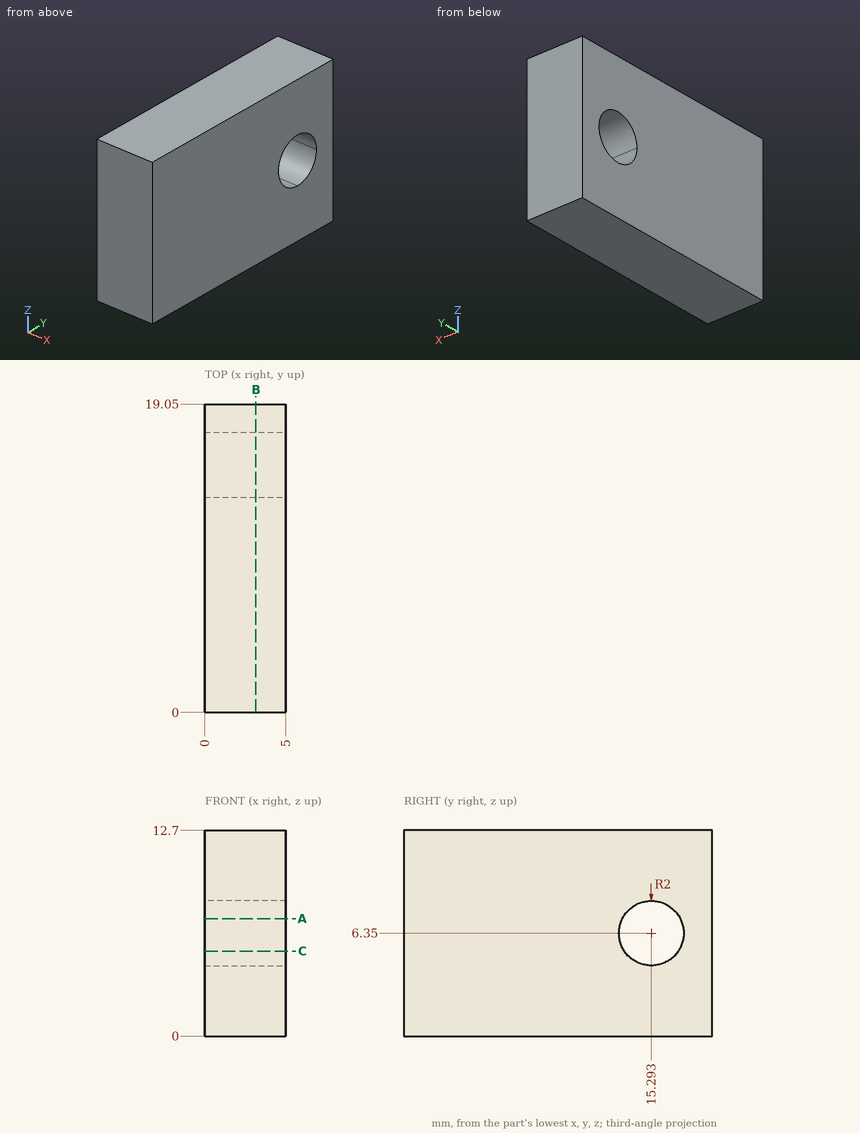
Source: three-view drawing plus pictorial views. Frame: mm from the lowest corner of the part. Coordinates: 2 decimals unless noted, no trailing zeros. Order: outer loops, then holes, each group sorted by start corner. A loop starts at its lowest first (then second) coordinate and runs counter-clockwise, first axis right, second up. Notation, with made-up numbers: M -16.75,83.5 L 0.25,83.5 A30 ccw 0.25,113.5 Z; hole C 19.5,10 d2. An arc over 180 degrees is marked long. One line per question, with ' | ' between items. Start each with the question number.
Item 1: Ray query, probe 1 along Y at (x, z) = (0.35, 6); probe 2 along Y at (x, z) = (1.35, 5.25); probe 3 along Z at (x, y) = (2.3, 14.5). Return the intervals inside material, ascending. Write a range as [from, to].
Item 2: Pin query (flat end, axial travel): pin 1 Ø1 at (x, y) = (2, 5.5) entering from -Z. Return the tip coordinate at first contact, or that it passes through.
Item 3: Cut plane C-C, the plane z = 5.25. Return the cut outline in (x, y).
Item 4: Cut plane B-B, the plane x = 3.15. Return the cut outline in (y, z), then the cut area to 3 significant figures.
Item 5: Cut plane A-A, the plane z = 7.25. Return the cut outline in (x, y), then the cut area to 3 significant figures.
A:
1) probe 1: y = [0, 13.32], [17.26, 19.05] | probe 2: y = [0, 13.62], [16.96, 19.05] | probe 3: z = [0, 4.51], [8.19, 12.7]
2) pin 1: stops at z = 0
3) outline: M 0,0 L 5,0 L 5,13.62 L 0,13.62 Z; M 0,16.96 L 5,16.96 L 5,19.05 L 0,19.05 Z
4) outline: M 0,0 L 19.05,0 L 19.05,12.7 L 0,12.7 Z; hole C 15.29,6.35 d4 | area: 229 mm2
5) outline: M 0,0 L 5,0 L 5,13.51 L 0,13.51 Z; M 0,17.08 L 5,17.08 L 5,19.05 L 0,19.05 Z | area: 77.4 mm2
